from build123d import *

# Parameters (mm, degrees)
EXTRUDE_DEPTH    = 2.8
EXTRUDE001_DEPTH = 2.8
SKETCH_W         = 68
SKETCH_H         = 40
SKETCH_R         = 5
PAD_DEPTH        = 8.5
SKETCH001_R      = 7.5
POCKET_DEPTH     = 4
SKETCH002_R      = 1.6
POCKET001_DEPTH  = 10
SKETCH003_R      = 1.6
PAD001_DEPTH     = 6
SKETCH004_W      = 11.5
SKETCH004_H      = 10
SKETCH004_R      = 1.6
PAD002_DEPTH     = 6


with BuildPart() as extrude_body:
    # Fusion → Extrude (new body)
    with BuildSketch(Plane.XY):
        Polygon((12.624044, -45.3857), (12.624044, -40.3857), (12.624044, -37.0857), (9.76616, -35.4357), (6.908276, -37.0857), (6.908276, -40.3857), (6.908276, -45.3857), align=None)
    extrude(amount=EXTRUDE_DEPTH)


with BuildPart() as extrude_body_1:
    # Extrude placement: moved
    add(extrude_body.part.moved(Location((13.2338, 33.7357, 9))))


with BuildPart() as extrude001:
    # Fusion001 → Extrude001 (new body)
    with BuildSketch(Plane.XY):
        Polygon((12.624044, -45.3857), (12.624044, -40.3857), (12.624044, -37.0857), (9.76616, -35.4357), (6.908276, -37.0857), (6.908276, -40.3857), (6.908276, -45.3857), align=None)
    extrude(amount=EXTRUDE001_DEPTH)


with BuildPart() as extrude001_1:
    # Extrude001 placement: moved
    add(extrude001.part.moved(Location((41.2338, 33.7357, 9))))


with BuildPart() as pad002:
    # Sketch → Pad (new body)
    with BuildSketch(Plane.XZ.offset(8.5)):
        with Locations((40, 23.5)):
            Rectangle(SKETCH_W, SKETCH_H)
        with Locations((15, 25.5)):
            Circle(SKETCH_R, mode=Mode.SUBTRACT)
        with Locations((32, 25.5)):
            Circle(SKETCH_R, mode=Mode.SUBTRACT)
        with Locations((49, 25.5)):
            Circle(SKETCH_R, mode=Mode.SUBTRACT)
        with Locations((66, 25.5)):
            Circle(SKETCH_R, mode=Mode.SUBTRACT)
    extrude(amount=-PAD_DEPTH)

    # Sketch001 → Pocket (cut)
    with BuildSketch(Plane(origin=(0, 0, 0), x_dir=(1, 0, 0), z_dir=(0, 1, 0))):
        with Locations((15, -25.5)):
            Circle(SKETCH001_R)
        with Locations((32, -25.5)):
            Circle(SKETCH001_R)
        with Locations((49, -25.5)):
            Circle(SKETCH001_R)
        with Locations((66, -25.5)):
            Circle(SKETCH001_R)
    extrude(amount=-POCKET_DEPTH, mode=Mode.SUBTRACT)

    # Sketch002 → Pocket001 (cut)
    with BuildSketch(Plane(origin=(0, -8.5, 3.5), x_dir=(1, 0, 0), z_dir=(0, 0, -1))):
        with Locations((51, -3.5)):
            Circle(SKETCH002_R)
        with Locations((23, -3.5)):
            Circle(SKETCH002_R)
    extrude(amount=-POCKET001_DEPTH, mode=Mode.SUBTRACT)

    # Cut: cut Extrude001
    add(extrude001_1.part, mode=Mode.SUBTRACT)

    # Cut001: cut Extrude body
    add(extrude_body_1.part, mode=Mode.SUBTRACT)

    # Sketch003 → Pad001 (new body)
    with BuildSketch(Plane.XY.offset(43.5)):
        Polygon((74, 0), (82.5, 36), (82.5, 46), (59.5, 46), (59.5, 36), (51, 0), align=None)
        with Locations((64.5, 43)):
            Circle(SKETCH003_R, mode=Mode.SUBTRACT)
        with Locations((77.5, 43)):
            Circle(SKETCH003_R, mode=Mode.SUBTRACT)
    extrude(amount=-PAD001_DEPTH)

    # Sketch004 → Pad002 (new body)
    with BuildSketch(Plane(origin=(0, 0, 37.5), x_dir=(1, 0, 0), z_dir=(0, 0, -1))):
        with Locations((65.25, -41)):
            Rectangle(SKETCH004_W, SKETCH004_H)
        with Locations((64.5, -43)):
            Circle(SKETCH004_R, mode=Mode.SUBTRACT)
    extrude(amount=PAD002_DEPTH)


solid = pad002.part
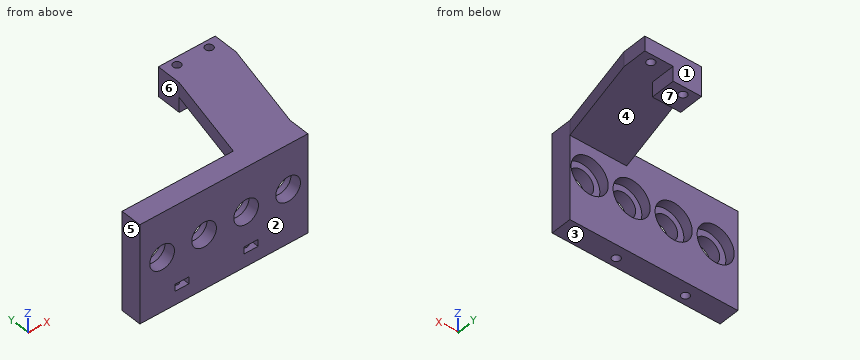
Geometry check sheet. Reference: the model listing, model coordinates, mm. Face numbers are marked on the shaded views. A direction names the side the tool comes from. Coordinates: 2 decimals unless noted, no trailing zeros. Order: outer loops, then holes, each group sorted by start corner. A loop starts at its lowest first (then second) coordinate and runs counter-clockwise, first axis right, second up. Notation, with made-up numbers: M -10.75,18.25 L 17.25,18.25 A34 ccw 17.25,54.25 Z; hole C 41.5,74 d9. An arc over 180 degrees is marked long. Use CSV: the item, a comma, the result in double quotes.
Item 1: Tool access check on the marked faces 5, 6 and 7. Record the directions out of +Z, -Z, +X, -X, +Y, -Y that give a thin tool (end or side, any length) a straight path to the whole face; none if there is none.
Returned:
face 5,"+Z, -Z, -X, +Y, -Y"
face 6,"+Z, -Z, -X, +Y"
face 7,"-Z, +X, -X, +Y"
Item 2: Cross-section at C-C on x = 77.5. Record the cut outline in (y, z).
Returned:
outline,"M 14.82,37.5 L 41.4,37.5 L 41.4,43.5 L 14.82,43.5 Z; M 44.6,37.5 L 46,37.5 L 46,43.5 L 44.6,43.5 Z"
Item 3: Cross-section at A-A on y = 43. Record the cut outline in (x, z).
Returned:
outline,"M 59.5,31.5 L 62.9,31.5 L 62.9,43.5 L 59.5,43.5 Z; M 66.1,31.5 L 71,31.5 L 71,37.5 L 75.9,37.5 L 75.9,43.5 L 66.1,43.5 Z; M 79.1,37.5 L 82.5,37.5 L 82.5,43.5 L 79.1,43.5 Z"
Item 4: Gauge pin test, flat ends, axial feed: pin 1 Ø11 at (x, y) = (64.5, 39) entering from -Z; pin 2 Ø12 at (x, z) = (33, 22.5) entering from +Y; pin 3 Ø7.5 at (x, z) = (68, 24.5) entering from +Y; pin 4 Ø12 at (x, z) = (66, 25.5) entering from -Y. Record the tip position at first contact, or that the pin passes through.
Returned:
pin 1,"stops at z = 31.5"
pin 2,"stops at y = 0"
pin 3,"stops at y = -4"
pin 4,"stops at y = -8.5"
Item 5: Cross-section at D-D on y = -5. Give the number of separate pieces and of enclosed holes in the cut face, then the cut area to 3 significant figures.
Returned:
separate pieces,"1"
enclosed holes,"4"
area,"2,330 mm2"
Item 6: Mould release check, pull along Y, two halves, no side actions. Record for the marked faces 1, 2, 3 and 4: pulls with the +Y half, pulls with the -Y half, needs draft (parallel to the pull), parting line crosses it, or undercut.
Returned:
face 1,"pulls with the +Y half"
face 2,"pulls with the -Y half"
face 3,"needs draft"
face 4,"undercut"
Item 7: Cross-section at B-B on z = 19.5. Record the cut outline in (x, y).
Returned:
outline,"M 6,-8.5 L 74,-8.5 L 74,0 L 70.5,0 L 70.5,-4 L 61.5,-4 L 61.5,0 L 53.5,0 L 53.5,-4 L 44.5,-4 L 44.5,0 L 36.5,0 L 36.5,-4 L 27.5,-4 L 27.5,0 L 19.5,0 L 19.5,-4 L 10.5,-4 L 10.5,0 L 6,0 Z"
Item 8: Thickness scan on line 1 along X through (y, z) = (-1.3, 25.5); line 2 along Y through (x, z) = (60, 35.5); line 3 along Z through (x, y) = (15, -2.55). Record the ranges inside material, lowest first.
Returned:
line 1,"x = 6 to 7.5, 22.5 to 24.5, 39.5 to 41.5, 56.5 to 58.5, 73.5 to 74"
line 2,"y = -8.5 to 0, 36 to 46"
line 3,"z = 3.5 to 18, 33 to 43.5"
